Build history of the part. All positions in model axes, mm. Face numbers are marked on the shaded views. A direction names the side the tool comes from. Coordinates: 2 decimals unless noted, no trailing zeros. Order: outer loops, then holes, each group sorted by start corner. A loop starts at its lowest first (then second) coordinate and runs counter-clockwise, first axis right, second up. Notation, with made-up numbers: (-30.5, 66.5) - (-14.5, 66.5) arc R37 cw to (-14.5, 102.5) - close; hole circle Ø10 at (39, 4.25). An arc over 180 degrees is marked (long way). Return JSON: item names as keys, results as strings.
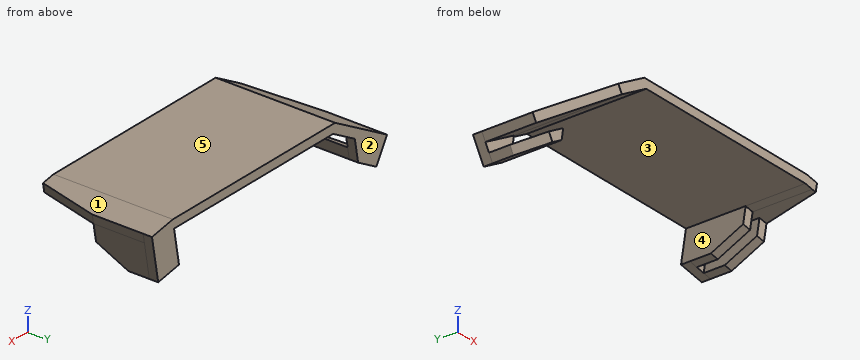
from build123d import *

# Parameters (mm, degrees)
BOSS_EXTRUDE1_DEPTH = 2
BOSS_EXTRUDE2_DEPTH = 25
BOSS_EXTRUDE3_DEPTH = 11.5
CUT_EXTRUDE2_DEPTH  = 2
CUT_EXTRUDE3_DEPTH  = 2.03188945
SKETCH8_W           = 7.96811055
SKETCH8_H           = 13.5
CUT_EXTRUDE4_DEPTH  = 2
CUT_EXTRUDE5_REACH  = 73.825
CUT_EXTRUDE6_DEPTH  = 2


with BuildPart() as part:
    # Sketch2 → Boss-Extrude1 (new body)
    with BuildSketch(Plane(origin=(0, 0, 0), x_dir=(1, 0, 0), z_dir=(0, 1, 0))):
        Polygon((-22.485232694, 2), (22.666829492, 2), (21.260674764, 9.843055182), (27.166507873, 10.901891943), (28.931235809, 1.058836761), (23.0254027, 0), (-23.0254027, 0), (-37.76942689, 8.590954614), (-34.748752683, 13.775115813), (-29.564591484, 10.754441606), (-28.637765281, 5.584918712), align=None)
    extrude(amount=-BOSS_EXTRUDE1_DEPTH)

    # Sketch3 → Boss-Extrude2 (add)
    with BuildSketch(Plane.XZ.offset(2)):
        Polygon((-37.76942689, -8.590954614), (-23.0254027, 0), (23.0254027, 0), (28.931235809, -1.058836761), (28.572662601, -3.058836759), (24.635440529, -2.352945585), (23.229285801, -10.196000769), (21.260674764, -9.843055182), (22.666829492, -2), (-22.485232694, -2), (-28.637765281, -5.584918712), (-36.762535488, -10.319008347), align=None)
    extrude(amount=BOSS_EXTRUDE2_DEPTH)

    # Sketch4 → Boss-Extrude3 (add)
    with BuildSketch(Plane.XZ.offset(2)):
        Polygon((25.197896837, -10.548946356), (26.604051565, -2.705891172), (28.572662601, -3.058836759), (27.166507873, -10.901891943), align=None)
        Polygon((-34.748752683, -13.775115813), (-35.755644085, -12.04706208), (-29.101178382, -8.169680159), (-29.564591484, -10.754441606), align=None)
    extrude(amount=BOSS_EXTRUDE3_DEPTH)

    # Sketch5 → Cut-Extrude2 (cut)
    with BuildSketch(Plane(origin=(-5.835962708, 0, 10.015834002), x_dir=(0.8640268665049071, 0, 0.5034457011016299), z_dir=(-0.5034457011016299, 0, 0.8640268665049071))):
        Polygon((-28.426722639, -27), (-36.958878734, -13.5), (-36.958878734, -27), align=None)
    extrude(amount=-CUT_EXTRUDE2_DEPTH, mode=Mode.SUBTRACT)

    # Sketch6 → Cut-Extrude3 (cut)
    with BuildSketch(Plane(origin=(0.717071985, 0, 3.999584852), x_dir=(0.9843055181910936, 0, -0.1764727935364628), z_dir=(0.1764727935364628, 0, 0.9843055181910936))):
        Polygon((25.664030936, -27), (28.664030936, -27), (28.664030936, -13.5), align=None)
    extrude(amount=-CUT_EXTRUDE3_DEPTH, mode=Mode.SUBTRACT)

    # Sketch8 → Cut-Extrude4 (cut)
    with BuildSketch(Plane(origin=(24.276941751, 0, -4.352530439), x_dir=(-0.17647279353646367, 0, -0.9843055181910934), z_dir=(0.9843055181910934, 0, -0.17647279353646367))):
        with Locations((1.952587588, -20.25)):
            Rectangle(SKETCH8_W, SKETCH8_H)
    extrude(amount=-CUT_EXTRUDE4_DEPTH, mode=Mode.SUBTRACT)

    # Cut-Extrude5: up to this face of the body (flat: up to its plane)
    cut_extrude5_end = Plane(part.part.faces().sort_by_distance((21.963752128, -6.75, -5.921527591))[0])
    # Sketch9 → Cut-Extrude5 (cut, up to the picked face)
    with BuildSketch(Plane(origin=(28.214163824, 0, -5.058421613), x_dir=(-0.17647279353646197, 0, -0.9843055181910936), z_dir=(0.9843055181910936, 0, -0.17647279353646197)), mode=Mode.PRIVATE) as cut_extrude5_sk1:
        Polygon((1.952587588, -13.5), (5.936642863, -6.75), (5.936642863, -13.5), align=None)
    cut_extrude5_tool1 = split(extrude(cut_extrude5_sk1.sketch, amount=-CUT_EXTRUDE5_REACH, mode=Mode.PRIVATE), bisect_by=cut_extrude5_end, keep=Keep.BOTH, mode=Mode.PRIVATE)
    add(cut_extrude5_tool1.solids().sort_by(Axis((27.400867, -11.25, -9.594716), (-0.9843055181910936, 0, 0.17647279353646197)))[0], mode=Mode.SUBTRACT)

    # Sketch10 → Cut-Extrude6 (cut)
    with BuildSketch(Plane(origin=(-2.815288501, 0, 4.831672803), x_dir=(-0.8640268665049072, 0, -0.5034457011016296), z_dir=(0.5034457011016296, 0, -0.8640268665049072))):
        Polygon((36.958878734, -6.75), (33.958878734, -13.5), (36.958878734, -13.5), align=None)
    extrude(amount=-CUT_EXTRUDE6_DEPTH, mode=Mode.SUBTRACT)


solid = part.part
1. Cut at A-A on y = -9. Give the cut face in (x, z), plus the area to 3 significant figures.
Check values:
{"outline": "(-37.77, -8.59) - (-36.76, -10.32) - (-22.49, -2) - (22.67, -2) - (21.5, -8.54) - (23.46, -8.89) - (24.64, -2.35) - (26.6, -2.71) - (25.43, -9.24) - (27.4, -9.59) - (28.93, -1.06) - (23.03, 0) - (-23.03, 0) - close; (-34.89, -11.54) - (-33.88, -13.27) - (-29.56, -10.75) - (-29.1, -8.17) - close", "area": "175 mm²"}
2. Cut at D-D on y = -23.25. Give the cut face in (x, z), plus the area to 3 significant figures.
Check values:
{"outline": "(-32.45, -5.49) - (-31.44, -7.22) - (-22.49, -2) - (22.67, -2) - (26.44, -2.68) - (26.8, -0.68) - (23.03, 0) - (-23.03, 0) - close", "area": "120 mm²"}
3. Cut at B-B on y = -18. Give the cut face in (x, z).
Check values:
{"outline": "(-35.31, -7.16) - (-34.31, -8.89) - (-22.49, -2) - (22.67, -2) - (27.59, -2.88) - (27.95, -0.88) - (23.03, 0) - (-23.03, 0) - close"}
4. Tool access for the marked faces 4 and 5: list every direction of +Z, -Z, +X, -X, +Y, -Y with a clear straight run to the whole face (end or side of a thin tool).
Check values:
{"face 4": "+Y, -Y", "face 5": "+Z, +X, -X, +Y, -Y"}
5. Probe L1, parallel to X at y = -3.75, z = -6; L2, parallel to Z at x = 0, y = -11.75; L3, parallel to X at y = -6.75, z = -6.25. List the from-to ranges inside material, lowest first.
Check values:
{"L1": "-33.32 to -29.35, 21.95 to 23.98, 26.01 to 28.05", "L2": "-2 to 0", "L3": "-33.75 to -29.78, 21.9 to 23.94, 25.97 to 28"}
6. Mould opens along X. For the marked faces 1, 2 and 3 say: pulls with the +X half, pulls with the -X half, needs draft (parallel to the pull), parting line crosses it, or undercut.
Check values:
{"face 1": "pulls with the +X half", "face 2": "needs draft", "face 3": "undercut"}
7. Cut at C-C on x = -3. Give the cut face in (y, z), plus the area to 3 significant figures.
Check values:
{"outline": "(-27, -2) - (0, -2) - (0, 0) - (-27, 0) - close", "area": "54.0 mm²"}
8. Drop flat-ended pins along their axis: pin 1 (2 mm diameter, centred on y = -3, z = -11, fed in from -X); pin 2 (3 mm diameter, centred on y = -14.5, z = -5, fed in from -X); pin 3 (1.5 mm diameter, centred on y = -14, z = -6, fed in from -X). Give the stop position or say it passes through.
Check values:
{"pin 1": "x = -36.95", "pin 2": "x = -34.18", "pin 3": "x = -34.61"}
